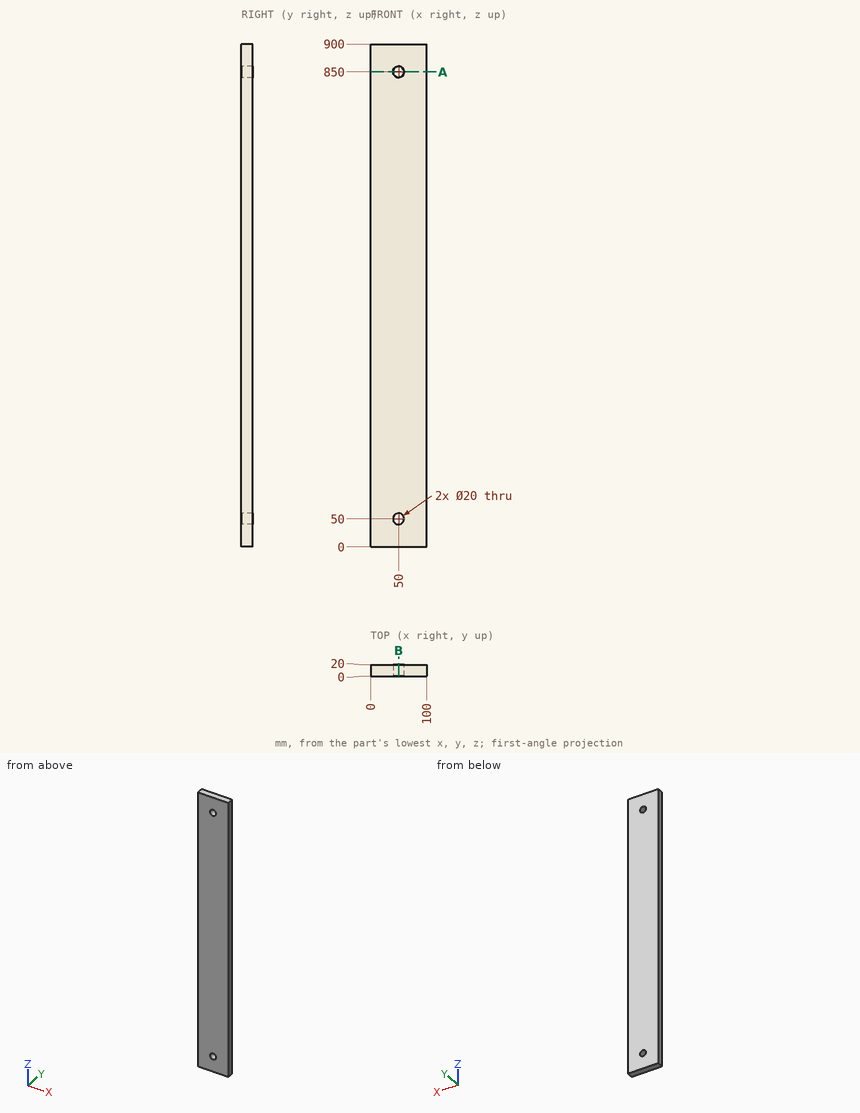
Study the drawing (mm; zero at the part's minimum x, y, z) and answer. Give positions to 0.01 mm unless a question says otherwise; leave off trailing zeros. Order: outer loops, then holes, each group sorted by start corner. A loop starts at its lowest first (then second) coordinate and runs counter-clockwise, first axis right, second up.
1) Consider line 1 along Z through (x, y) = (50, 9.5); line 2 along X through (y, z) = (11.25, 850); line 3 along Z through (x, y) = (58, 10). Determine where each line is inside the solid, lowest interval first.
Reported:
line 1: z = 0 to 40, 60 to 840, 860 to 900
line 2: x = 0 to 40, 60 to 100
line 3: z = 0 to 44, 56 to 844, 856 to 900
2) Find section B-B on x = 50. Write down the section's boundary in (y, z), then the cut area to 3 significant figures.
Reported:
outline: (0, 0) - (20, 0) - (20, 40) - (0, 40) - close; (0, 60) - (20, 60) - (20, 840) - (0, 840) - close; (0, 860) - (20, 860) - (20, 900) - (0, 900) - close
area: 17,200 mm2
3) Find section A-A on z = 850. Write down the section's boundary in (x, y).
Reported:
outline: (0, 0) - (40, 0) - (40, 20) - (0, 20) - close; (60, 0) - (100, 0) - (100, 20) - (60, 20) - close
